```python
from build123d import *

# Parameters (mm, degrees)
F1_DEPTH = 38.1
F0_W     = 152.4
F0_H     = 38.1
F0_W_2   = 38.1
F2_DEPTH = 38.1


with BuildPart() as f1:
    # F0 (on Front) → F1 (new body)
    with BuildSketch(Plane.XZ):
        Polygon((-190.5, 31.534294), (-152.4, 31.534294), (166.608291, 262.161064), (166.608291, 300.261064), align=None)
    extrude(amount=F1_DEPTH)

    # F0 (on Front) → F2 (join)
    with BuildSketch(Plane.XZ):
        with Locations((-76.2, 12.484294)):
            Rectangle(F0_W, F0_H)
        with Locations((-171.45, 12.484294)):
            Rectangle(F0_W_2, F0_H)
        Polygon((0, 31.534294), (0, -6.565706), (166.608291, 109.761064), (166.608291, 147.861064), align=None)
        Polygon((-190.5, 31.534294), (-152.4, 31.534294), (166.608291, 262.161064), (166.608291, 300.261064), align=None)
        Polygon((166.608291, 147.861064), (166.608291, 109.761064), (204.708291, 109.761064), (204.708291, 262.161064), (166.608291, 262.161064), align=None)
        with Locations((185.658291, 281.211064)):
            Rectangle(F0_W_2, F0_H)
    extrude(amount=F2_DEPTH)


solid = f1.part
```
Design review of the part built by this model. Coordinates are the model's own, in mm. A direction names the side the tool comes from. Round coordinates to 2 decimals unless told otherwise and drop trailing zeros. Write each loop counter-clockwise with the first axis right and the second up, starting at its lowest first coordinate (ties: lowest second). Pieces come first, ordered by that corner, then holes. Notation, with made-up numbers: (80, 1.25) -> (103, 1.25) arc R13 cw to (103, 24.25) -> close; hole circle Ø9 at (33, -25). An arc over 180 degrees is marked (long way). Answer in a Markdown table with one row per item.
Q1. Take a section at D-D, the plane z = 275.5. State the section outline as (x, y) points.
The answers:
| item | result |
|---|---|
| outline | (133.7, -38.1) -> (204.71, -38.1) -> (204.71, 0) -> (133.7, 0) -> close |
Q2. Clearance check with flat-ended pins moving along their axes: pin 1 Ø5 at (x, y) = (-145.5, -30) entering from +Z; pin 2 Ø3 at (x, z) = (107.5, 240.5) entering from +Y; pin 3 Ø11.5 at (x, y) = (-46.5, -26) entering from +Z; pin 4 Ø2 at (y, z) = (-16, 103.5) entering from +X. State where each tip first meets the part, or that it passes through.
The answers:
| item | result |
|---|---|
| pin 1 | z = 67.28 |
| pin 2 | y = 0 |
| pin 3 | z = 144.22 |
| pin 4 | x = 159.07 |
Q3. For faces 1 (the face through (204.708, -19, 204)), 2 (the face through (166.608, -19, 206)), list the 3-axis set-ups (+Z, -Z, +X, -X, +Y, -Y) from which the entire face can be reached by the end or side of a thin tool; tool diameter is ignored.
The answers:
| item | result |
|---|---|
| face 1 | +Z, -Z, +X, +Y, -Y |
| face 2 | +Y, -Y |
Q4. Take a section at C-C, the plane y = -18. State the section outline as (x, z) points.
The answers:
| item | result |
|---|---|
| outline | (-190.5, -6.57) -> (0, -6.57) -> (166.61, 109.76) -> (204.71, 109.76) -> (204.71, 300.26) -> (166.61, 300.26) -> (-190.5, 31.53) -> close; hole (-152.4, 31.53) -> (0, 31.53) -> (166.61, 147.86) -> (166.61, 262.16) -> close |
Q5. To check wall thickness, follow L1, parallel to Z at x = 10.5, y = -10.5; L2, parallel to X at y = -5.5, z = 50; L3, parallel to Z at x = 62.5, y = -13. State the ranges of each line that lie inside material, in increasing order. Write a range as [from, to].
The answers:
| item | result |
|---|---|
| L1 | [0.77, 38.87], [149.3, 182.79] |
| L2 | [-165.96, -126.86], [26.45, 81.02] |
| L3 | [37.07, 75.17], [186.9, 221.92] |
Q6. Take a section at B-B, the plane z = 180. State the section outline as (x, y) points, then the cut area to 3 significant figures.
The answers:
| item | result |
|---|---|
| outline | (6.79, -38.1) -> (52.96, -38.1) -> (52.96, 0) -> (6.79, 0) -> close; (166.61, -38.1) -> (204.71, -38.1) -> (204.71, 0) -> (166.61, 0) -> close |
| area | 3,210 mm² |
Q7. Take a section at A-A, the plane x = -27. State the section outline as (y, z) points, then the cut area to 3 significant figures.
The answers:
| item | result |
|---|---|
| outline | (-38.1, -6.57) -> (0, -6.57) -> (0, 31.53) -> (-38.1, 31.53) -> close; (-38.1, 122.19) -> (0, 122.19) -> (0, 154.57) -> (-38.1, 154.57) -> close |
| area | 2,690 mm² |
Q8. Draft analysis for pull direction Z (two halves, no side actions). For faces 3 (the face through (185, -19, 300.261)), 4 (the face through (185, -19, 109.761)), 5 (the face through (84.47, -18.78, 90.51)), 6 (the face through (21, -38.1, 159)), state which applies: +Z half, -Z half, draft (parallel to the pull), parting line (faces both ways), or undercut.
The answers:
| item | result |
|---|---|
| face 3 | +Z half |
| face 4 | -Z half |
| face 5 | undercut |
| face 6 | draft |
